from build123d import *

# Parameters (mm, degrees)
SKETCH1_R           = 2.35
SKETCH1_R_2         = 0.5
BOSS_EXTRUDE1_DEPTH = 1


with BuildPart() as part:
    # Sketch1 → Boss-Extrude1 (new body)
    with BuildSketch(Plane(origin=(0, 0, 0), x_dir=(1, 0, 0), z_dir=(0, 1, 0))):
        with BuildLine():
            Line((1.320293399, 4.30195599), (0, 4.5))
            ThreePointArc((0, 4.5), (-4.5, 0), (0, -4.5))
            Line((0, -4.5), (1.320293399, -4.30195599))
            Line((1.320293399, -4.30195599), (15, -2.25))
            ThreePointArc((15, -2.25), (17.25, 0), (15, 2.25))
            Line((15, 2.25), (1.320293399, 4.30195599))
        make_face()
        Circle(SKETCH1_R, mode=Mode.SUBTRACT)
        with Locations((15, 0)):
            Circle(SKETCH1_R_2, mode=Mode.SUBTRACT)
    extrude(amount=BOSS_EXTRUDE1_DEPTH)


solid = part.part
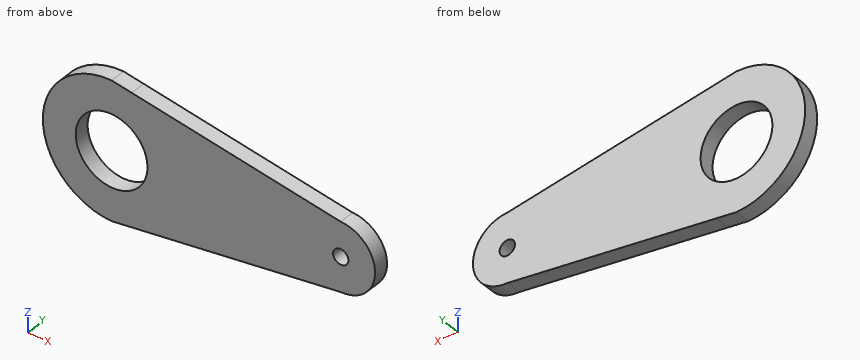
Source: CAD feature listing. Evaluate the final solid. Frame: model axes, mm. Round coordinates to 2 decimals unless told otherwise and drop trailing zeros. Write each loop counter-clockwise with the first axis right and the second up, starting at its lowest first coordinate (ties: lowest second). Pieces come first, ordered by that corner, then holes. Notation, with made-up numbers: (-25, 80.5) - (13, 80.5) arc R18 ccw to (13, 93.5) - close; hole circle Ø5 at (-37.75, 38.25). An arc over 180 degrees is marked (long way). Use CSV: the item, a comma, the result in double quotes. Start each with the question number.
(1) Material intervals for probe 1 along X at (y, z) = (0.55, 0); probe 2 along Z at (x, y) = (15, 0.65); probe 3 along X at (y, z) = (0.65, 0.25), sorted ascending. Write a range as [from, to].
(2) Cut plane B-B, the plane y = 0.35. Return loops of the section in (x, z), and give its area (3 significant figures).
(3) Cut plane D-D, the plane z = 1. Return loops of the section in (x, y).
(4) Cut plane C-C, the plane x = -1.75. Return loops of the section in (y, z), and give its area (3 significant figures).
(5) First-contact query: pin 1 Ø4 at (x, z) = (0, 0) entering from +Y; pin 2 Ø1.5 at (x, z) = (1.5, -1) entering from -Y. Flat tips, straight axial feed; report the tip coordinate or a pass-through.
(6) Cut plane A-A, the plane z = 0. Return loops of the section in (x, y), and give its area (4 significant figures).
Geometry says:
1,probe 1,"[-4.5, -2.35], [2.35, 14.5], [15.5, 17.25]"
1,probe 2,"[-2.25, -0.5], [0.5, 2.25]"
1,probe 3,"[-4.49, -2.34], [2.34, 14.57], [15.43, 17.24]"
2,outline,"(0, -4.5) - (15, -2.25) arc R2.25 ccw to (15, 2.25) - (0, 4.5) arc R4.5 ccw to start; hole circle Ø4.7 at (0, 0); hole circle Ø1 at (15, 0)"
2,area,"123 mm²"
3,outline,"(-4.39, 0) - (-2.13, 0) - (-2.13, 1) - (-4.39, 1) - close; (2.13, 0) - (17.02, 0) - (17.02, 1) - (2.13, 1) - close"
4,outline,"(0, -4.15) - (1, -4.15) - (1, -1.57) - (0, -1.57) - close; (0, 1.57) - (1, 1.57) - (1, 4.15) - (0, 4.15) - close"
4,area,"5.15 mm²"
5,pin 1,"through"
5,pin 2,"y = 0"
6,outline,"(-4.5, 0) - (-2.35, 0) - (-2.35, 1) - (-4.5, 1) - close; (2.35, 0) - (14.5, 0) - (14.5, 1) - (2.35, 1) - close; (15.5, 0) - (17.25, 0) - (17.25, 1) - (15.5, 1) - close"
6,area,"16.05 mm²"
